The model under review builds one solid part; all positions refer to its coordinate system, in mm. Give positions to 0.01 mm unless a question says otherwise; leave off trailing zeros. Order: outer loops, then holes, each group sorted by start corner. A loop starts at its lowest first (then second) coordinate and runs counter-clockwise, first axis right, second up. Notation, with made-up numbers: (33.5, 7.25) -> (69.5, 7.25) arc R14 cw to (69.5, 26.25) -> close; hole circle Ø8 at (67.25, 26.25). An arc over 180 degrees is marked (long way). Use one line per item in the form item = value.
```python
from build123d import *

# Parameters (mm, degrees)
CYLINDER004_R          = 1.75
CYLINDER004_DEPTH      = 6
ARRAY004_X_COUNT       = 2
ARRAY004_X_PITCH       = 22
ARRAY004_Y_COUNT       = 2
ARRAY004_Y_PITCH       = 40
BOX011_W               = 20
BOX011_H               = 20
BOX011_DEPTH           = 20
BOX011_PLACEMENT_ANGLE = 45
BOX012_W               = 20
BOX012_H               = 20
BOX012_DEPTH           = 20
BOX012_PLACEMENT_ANGLE = 45
BOX009_W               = 20
BOX009_H               = 20
BOX009_DEPTH           = 20
BOX009_PLACEMENT_ANGLE = -45
BOX010_W               = 20
BOX010_H               = 20
BOX010_DEPTH           = 20
BOX010_PLACEMENT_ANGLE = -45
BOX008_W               = 128
BOX008_H               = 99
BOX008_DEPTH           = 20
CUT005_PLACEMENT_ANGLE = 180


with BuildPart() as array004:
    # Cylinder004 → Cylinder004 (new body)
    with BuildSketch(Plane.XY):
        Circle(CYLINDER004_R)
    extrude(amount=CYLINDER004_DEPTH)

    # Array004 X: Array004 ×2


with BuildPart() as array004_1:
    add(array004.part)
    with Locations(*[(i * ARRAY004_X_PITCH, 0, 0) for i in range(1, ARRAY004_X_COUNT)]):
        add(array004.part)

    # Array004 Y: Array004 ×2


with BuildPart() as array004_2:
    add(array004_1.part)
    with Locations(*[(0, i * ARRAY004_Y_PITCH, 0) for i in range(1, ARRAY004_Y_COUNT)]):
        add(array004_1.part)


with BuildPart() as array004_3:
    # Array004 placement: moved
    add(array004_2.part.moved(Location((37.5, -8, 0))))


with BuildPart() as cubo007:
    # Box011 → Box011 (new body)
    with BuildSketch(Plane.XY):
        with Locations((10, 10)):
            Rectangle(BOX011_W, BOX011_H)
    extrude(amount=BOX011_DEPTH)


with BuildPart() as cubo007_1:
    # Box011 placement: moved
    add(cubo007.part.moved(Location((-14, -28.65, 0))).rotate(Axis((-14, -28.65, 0), (0, 0, 1)), BOX011_PLACEMENT_ANGLE))


with BuildPart() as cubo008:
    # Box012 → Box012 (new body)
    with BuildSketch(Plane.XY):
        with Locations((10, 10)):
            Rectangle(BOX012_W, BOX012_H)
    extrude(amount=BOX012_DEPTH)


with BuildPart() as cubo008_1:
    # Box012 placement: moved
    add(cubo008.part.moved(Location((-14, 70.35, 0))).rotate(Axis((-14, 70.35, 0), (0, 0, 1)), BOX012_PLACEMENT_ANGLE))


with BuildPart() as cubo005:
    # Box009 → Box009 (new body)
    with BuildSketch(Plane.XY):
        with Locations((10, 10)):
            Rectangle(BOX009_W, BOX009_H)
    extrude(amount=BOX009_DEPTH)


with BuildPart() as cubo005_1:
    # Box009 placement: moved
    add(cubo005.part.moved(Location((100, -14.5, 0))).rotate(Axis((100, -14.5, 0), (0, 0, 1)), BOX009_PLACEMENT_ANGLE))


with BuildPart() as fusion005:
    # Box010 → Box010 (new body)
    with BuildSketch(Plane.XY):
        with Locations((10, 10)):
            Rectangle(BOX010_W, BOX010_H)
    extrude(amount=BOX010_DEPTH)


with BuildPart() as fusion005_1:
    # Box010 placement: moved
    add(fusion005.part.moved(Location((99.8, 84.5, 0))).rotate(Axis((99.8, 84.5, 0), (0, 0, 1)), BOX010_PLACEMENT_ANGLE))

    # Fusion005: union Cubo007, Cubo008, Cubo005
    add(cubo007_1.part)
    add(cubo008_1.part)
    add(cubo005_1.part)


with BuildPart() as obj1:
    # Box008 → Box008 (new body)
    with BuildSketch(Plane(origin=(-14, -14.5, 0), x_dir=(1, 0, 0), z_dir=(0, 0, 1))):
        with Locations((64, 49.5)):
            Rectangle(BOX008_W, BOX008_H)
    extrude(amount=BOX008_DEPTH)

    # Cut004: cut Fusion005
    add(fusion005_1.part, mode=Mode.SUBTRACT)

    # Cut005: cut Array004
    add(array004_3.part, mode=Mode.SUBTRACT)


with BuildPart() as obj1_1:
    # Cut005 placement: moved
    add(obj1.part.moved(Location((71, -33.7, -17))).rotate(Axis((71, -33.7, -17), (0, 1, 0)), CUT005_PLACEMENT_ANGLE))


solid = obj1_1.part
```
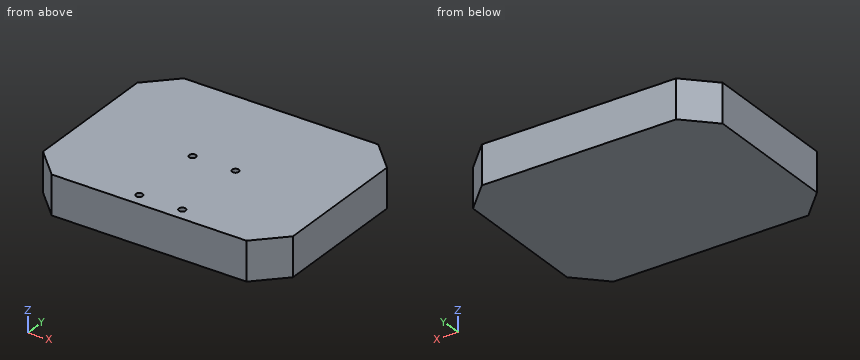
1. For L1, parallel to Y at x = 11.5, z = -21.7; L2, parallel to X at y = -3, z = -20; L3, parallel to Y at x = 75, z = -29.25, list the stretches that pass through material, from the lowest coordinate up.
Values:
L1 = -48.2 to -43.45, -39.95 to -3.45, 0.05 to 50.8
L2 = -43 to 10.33, 12.67 to 32.33, 34.67 to 85
L3 = -44.07 to 46.65
2. For pin 1 Ø1 at (x, y) = (11.5, -41.5) entering from +Z, flat-tipped, find the tip position at first contact; note if it passes through.
Values:
pin_1 = -23
3. Add section A-A on x = 11.5. Give the boundary of the cut face in (y, z).
Values:
outline = (-48.2, -37) -> (50.8, -37) -> (50.8, -17) -> (0.05, -17) -> (0.05, -23) -> (-3.45, -23) -> (-3.45, -17) -> (-39.95, -17) -> (-39.95, -23) -> (-43.45, -23) -> (-43.45, -17) -> (-48.2, -17) -> close
4. Add section D-D on y = 41. Give the boundary of the cut face in (x, z).
Values:
outline = (-38.6, -37) -> (80.65, -37) -> (80.65, -17) -> (-38.6, -17) -> close
5. Add section B-B on y = -1.7. Give the boundary of the cut face in (x, z).
Values:
outline = (-43, -37) -> (85, -37) -> (85, -17) -> (35.25, -17) -> (35.25, -23) -> (31.75, -23) -> (31.75, -17) -> (13.25, -17) -> (13.25, -23) -> (9.75, -23) -> (9.75, -17) -> (-43, -17) -> close
